from build123d import *

# Parameters (mm, degrees)
SKETCH_3_W               = 24
SKETCH_3_H               = 17.528375635
SKETCH_4_R               = 10.5
CUT_EXTRUDE_1_DEPTH      = 30
PATTERN_CIRCULAR_1_COUNT = 12


with BuildPart() as part:
    # 草图2 → 旋转1 (revolve)
    with BuildSketch(Plane.XY):
        with BuildLine():
            Line((628.514440138, -27.938395666), (628.514440138, -67.388903254))
            Line((628.514440138, -67.388903254), (628.514440138, -106.839410841))
            Line((628.514440138, -106.839410841), (644.137468569, -106.839410841))
            Line((644.137468569, -106.839410841), (644.137468569, -156.607948671))
            Line((644.137468569, -156.607948671), (660.065119858, -156.607948671))
            add(Edge.make_bspline(
                [(660.065119858, -156.607948671), (663.097961625, -156.988826471), (667.510654429, -158.674715159), (674.04876802, -164.83793422), (674.645699136, -171.621615989), (673.724213488, -175.886758841)],
                knots=[0, 0, 0, 0, 2126.071479581, 3119.447228311, 6154.527529927, 6154.527529927, 6154.527529927, 6154.527529927], degree=3, weights=[1, 1, 1, 1, 1, 1]))
            ThreePointArc((673.724213488, -175.886758841), (678.502301213, -187.396306093), (681.053033074, -199.594402961))
            Line((681.053033074, -199.594402961), (681.141679927, -199.594402961))
            Line((681.141679927, -199.594402961), (718.926959628, -199.594402961))
            Line((718.926959628, -199.594402961), (718.926959628, -189.098920651))
            ThreePointArc((718.926959628, -189.098920651), (720.464553406, -185.386840898), (724.176633159, -183.849247119))
            Line((724.176633159, -183.849247119), (732.610849344, -183.849247119))
            Line((732.610849344, -183.849247119), (732.610849344, -166.320871484))
            Line((732.610849344, -166.320871484), (715.675420917, -166.320871484))
            Line((715.675420917, -166.320871484), (715.675420917, -164.221002072))
            Line((715.675420917, -164.221002072), (701.57964043, -163.876181958))
            add(Edge.make_bspline(
                [(701.57964043, -163.876181958), (696.836978513, -162.873820387), (682.485210268, -157.676172339), (679.945843963, -129.423738671), (658.481699004, -105.854615848), (657.726950227, -82.12575596), (658.548500632, -70.985718628)],
                knots=[0, 0, 0, 0, 1057.430308103, 2997.111062824, 5402.743204918, 7834.148234872, 7834.148234872, 7834.148234872, 7834.148234872], degree=3, weights=[1, 1, 1, 1, 1, 1, 1]))
            Line((658.548500632, -70.985718628), (642.037599156, -70.985718628))
            Line((642.037599156, -70.985718628), (642.037599156, -67.835914509))
            Line((642.037599156, -67.835914509), (644.13666516, -67.835914509))
            Line((644.13666516, -67.835914509), (644.13666516, -27.938395666))
            Line((644.13666516, -27.938395666), (628.514440138, -27.938395666))
        make_face()
        Polygon((733.66078405, -166.320871484), (732.610849344, -166.320871484), (732.610849344, -183.849247119), (755.709412884, -183.849247119), (755.709412884, -166.320871484), (754.659478178, -166.320871484), align=None)
    revolve(axis=Axis((599.514440138, -67.388903254, 0), (0, -1, 0)))

    # 草图3 → 旋转2 (revolve)
    with BuildSketch(Plane.XY):
        with Locations((431.319467391, -175.085059301)):
            Rectangle(SKETCH_3_W, SKETCH_3_H)
    revolve(axis=Axis((599.514440138, -67.835914509, 0), (0, 1, 0)))

    # 草图4 → 切除-拉伸1 (cut)
    with BuildSketch(Plane(origin=(0, -166.320871484, 0), x_dir=(1, 0, 0), z_dir=(0, 1, 0))):
        with Locations((461.514440138, 0)):
            Circle(SKETCH_4_R)
    cut_extrude_1 = extrude(amount=-CUT_EXTRUDE_1_DEPTH, mode=Mode.SUBTRACT)

    # 阵列(圆周)1: 切除-拉伸1 ×12 about axis
    pattern_circular_1_axis = Axis((599.514440138, 0, 0), (0, 1, 0))
    for i in range(1, PATTERN_CIRCULAR_1_COUNT):
        add(cut_extrude_1.rotate(pattern_circular_1_axis, i * 360 / PATTERN_CIRCULAR_1_COUNT), mode=Mode.SUBTRACT)


solid = part.part
Check sheet for the modelled part. Datum: model origin and axes. Units: mm. A direction names the side the tool comes from. Round coordinates to 2 decimals unless told otherwise and drop trailing zeros. Loops run counter-clockwise (first coordinate to the right, second up) from the corner with the lowest first, then second, coordinate; pieces in that order, holes last.
1. Gauge pin test, flat ends, axial feed: pin 1 Ø12 at (x, y) = (560.5, -132) entering from -Z; pin 2 Ø8 at (y, z) = (-97.5, -28.5) entering from -X; pin 3 Ø24 at (x, z) = (668.51, -119.51) entering from +Y. Record the tip position at first contact, or that the pin passes through.
2. Scan lines: probe 1 along X at (y, z) = (-178.75, -69); probe 2 along X at (y, z) = (-174, 69); probe 3 along X at (y, z) = (-153, 14). Record each from-to range of solid material in increasing order.
3. Mould release check, pull along X, two halves, no side actions. Record for faces 4 (the cylindrical face through (480.217, -194.273, 5.25)), 5 (the cylindrical face through (678.214, -174.962, 123.533)), 6 (the flat face through (629, -27.938, 1)): released by +X, released by -X, zero draft, split by the parting line, or undercut.
4. Sectioned sample at A-A on z = -139.5. Record the boundary of the cut face in (x, y).
5. Sectioned sample at C-C on z = 0. Give the number of separate pieces and of enclosed holes in the cut face, and give its area (3 significant figures).
6. Set-up check for faces 1 (the cylindrical face through (708.776, -174.962, 66.724)), 2 (the conical face through (694.429, -163.893, -39.354)), 3 (the flat face through (570, -106.839, 1)): record each of +Z, -Z, +X, -X, +Y, -Y from which the full face is reachable in a straight line by a thin tool's end or side.
7. Sectioned sample at B-B on y = -52. Record the boundary of the cut face in (x, z), and give its area (3 significant figures).
Recorded:
1. pin 1: stops at z = -71.31
1. pin 2: stops at x = 543.82
1. pin 3: stops at y = -166.32
2. probe 1: x = 433.05 to 469.5, 490.5 to 568.52, 630.5 to 708.53, 729.53 to 765.98
2. probe 2: x = 433.05 to 469.5, 490.5 to 571.37, 627.66 to 708.53, 729.53 to 765.98
2. probe 3: x = 515.64 to 557.14, 641.88 to 683.39
3. face 4: split by the parting line
3. face 5: undercut
3. face 6: zero draft
4. outline: (485.45, -183.85) - (589.12, -183.85) - (589.12, -166.32) - (485.45, -166.32) - close; (609.91, -183.85) - (713.58, -183.85) - (713.58, -166.32) - (609.91, -166.32) - close
5. separate pieces: 4
5. enclosed holes: 0
5. area: 11,500 mm2
6. face 1: +Y, -Y
6. face 2: +Y
6. face 3: -Y
7. outline: circle Ø89.24 at (599.51, 0); hole circle Ø58 at (599.51, 0)
7. area: 3,610 mm2
